from build123d import *

# Parameters (mm, degrees)
SKETCH1_W           = 2.9718
SKETCH1_H           = 25.1968
BOSS_EXTRUDE1_DEPTH = 3.175


with BuildPart() as part:
    # Sketch1 → Boss-Extrude1 (new body)
    with BuildSketch(Plane(origin=(0, 0, 0), x_dir=(1, 0, 0), z_dir=(0, 1, 0))):
        Polygon((-137.987314286, 58.785125), (-151.391257143, 58.785125), (-151.391257143, 61.960125), (-164.294457143, 61.960125), (-164.294457143, 58.785125), (-177.6984, 58.785125), (-177.6984, 61.960125), (-190.6016, 61.960125), (-190.6016, 58.785125), (-203.3016, 58.785125), (-203.3016, -58.785125), (-190.6016, -58.785125), (-190.6016, -61.960125), (-177.6984, -61.960125), (-177.6984, -58.785125), (-164.294457143, -58.785125), (-164.294457143, -61.960125), (-151.391257143, -61.960125), (-151.391257143, -58.785125), (-137.987314286, -58.785125), (-137.987314286, -61.960125), (-125.084114286, -61.960125), (-125.084114286, -58.785125), (-111.680171429, -58.785125), (-111.680171429, -61.960125), (-98.776971429, -61.960125), (-98.776971429, -58.785125), (-85.373028571, -58.785125), (-85.373028571, -61.960125), (-72.469828571, -61.960125), (-72.469828571, -58.785125), (-59.065885714, -58.785125), (-59.065885714, -61.960125), (-46.162685714, -61.960125), (-46.162685714, -58.785125), (-32.758742857, -58.785125), (-32.758742857, -61.960125), (-19.855542857, -61.960125), (-19.855542857, -58.785125), (-6.4516, -58.785125), (-6.4516, -61.960125), (6.4516, -61.960125), (6.4516, -58.785125), (19.855542857, -58.785125), (19.855542857, -61.960125), (32.758742857, -61.960125), (32.758742857, -58.785125), (46.162685714, -58.785125), (46.162685714, -61.960125), (59.065885714, -61.960125), (59.065885714, -58.785125), (72.469828571, -58.785125), (72.469828571, -61.960125), (85.373028571, -61.960125), (85.373028571, -58.785125), (98.776971429, -58.785125), (98.776971429, -61.960125), (111.680171429, -61.960125), (111.680171429, -58.785125), (125.084114286, -58.785125), (125.084114286, -61.960125), (137.987314286, -61.960125), (137.987314286, -58.785125), (151.391257143, -58.785125), (151.391257143, -61.960125), (164.294457143, -61.960125), (164.294457143, -58.785125), (177.6984, -58.785125), (177.6984, -61.960125), (190.6016, -61.960125), (190.6016, -58.785125), (203.3016, -58.785125), (203.3016, 58.785125), (190.6016, 58.785125), (190.6016, 61.960125), (177.6984, 61.960125), (177.6984, 58.785125), (164.294457143, 58.785125), (164.294457143, 61.960125), (151.391257143, 61.960125), (151.391257143, 58.785125), (137.987314286, 58.785125), (137.987314286, 61.960125), (125.084114286, 61.960125), (125.084114286, 58.785125), (111.680171429, 58.785125), (111.680171429, 61.960125), (98.776971429, 61.960125), (98.776971429, 58.785125), (85.373028571, 58.785125), (85.373028571, 61.960125), (72.469828571, 61.960125), (72.469828571, 58.785125), (59.065885714, 58.785125), (59.065885714, 61.960125), (46.162685714, 61.960125), (46.162685714, 58.785125), (32.758742857, 58.785125), (32.758742857, 61.960125), (19.855542857, 61.960125), (19.855542857, 58.785125), (6.4516, 58.785125), (6.4516, 61.960125), (-6.4516, 61.960125), (-6.4516, 58.785125), (-19.855542857, 58.785125), (-19.855542857, 61.960125), (-32.758742857, 61.960125), (-32.758742857, 58.785125), (-46.162685714, 58.785125), (-46.162685714, 61.960125), (-59.065885714, 61.960125), (-59.065885714, 58.785125), (-72.469828571, 58.785125), (-72.469828571, 61.960125), (-85.373028571, 61.960125), (-85.373028571, 58.785125), (-98.776971429, 58.785125), (-98.776971429, 61.960125), (-111.680171429, 61.960125), (-111.680171429, 58.785125), (-125.084114286, 58.785125), (-125.084114286, 61.960125), (-137.987314286, 61.960125), align=None)
        with Locations((-198.4375, 25.4)):
            Rectangle(SKETCH1_W, SKETCH1_H, mode=Mode.SUBTRACT)
        with Locations((-198.4375, -25.4)):
            Rectangle(SKETCH1_W, SKETCH1_H, mode=Mode.SUBTRACT)
        with Locations((198.4375, 25.4)):
            Rectangle(SKETCH1_W, SKETCH1_H, mode=Mode.SUBTRACT)
        with Locations((198.4375, -25.4)):
            Rectangle(SKETCH1_W, SKETCH1_H, mode=Mode.SUBTRACT)
    extrude(amount=BOSS_EXTRUDE1_DEPTH)


solid = part.part
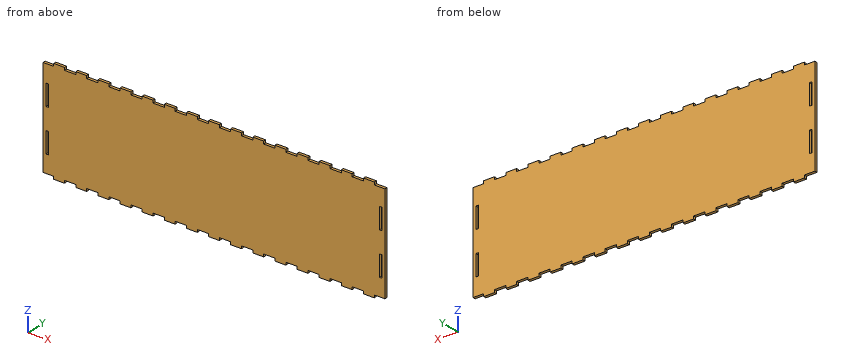
Source: CAD feature listing. Evaluate the final solid. Frame: model axes, mm. Round coordinates to 2 decimals unless told otherwise and drop trailing zeros. Loops run counter-clockwise (first coordinate to the right, second up) from the corner with the lowest first, then second, coordinate; pieces in that order, holes last. Notation, with made-up numbers: (65, -11.75) -> (112, -11.75) arc R14 ccw to (112, -4.75) -> close; hole circle Ø10 at (68.25, 40.25). An arc over 180 degrees is marked (long way). Answer as a JSON object with one key per item and string values. Group by question number.
Q1. Section query A-A (y = 1.75). State how many separate pieces and enclosed holes the cut face has, plus the area to 3 significant figures.
Q2. Contact query for flat-ended pins moving along their axis: P1, Ø1, axis at y = 1.5, z = 60, coming from the +X side; P2, Ø0.9, axis at x = -199, y = 2, coming from the -Z side; P3, Ø1.6, axis at x = 63.5, y = 2, coming from the +Z side. Output: stop coordinate, or through.
Q3. Section query B-B (x = -171.5). Output: boundary loops of the cut face in (y, z) (3 decimals).
Q4. Ray query, line 1 (X direction, y = 1.5, z = -25); line 2 (Z direction, x = 34, y = 3). Return the intervals inside material, ascending. Write a range as from..to.
Completed:
{
 "1": {"separate pieces": "1", "enclosed holes": "4", "area": "48,700 mm²"},
 "2": {"P1": "x = 190.6", "P2": "z = -58.79", "P3": "z = 58.79"},
 "3": {"outline": "(0, -58.785) -> (3.175, -58.785) -> (3.175, 58.785) -> (0, 58.785) -> close"},
 "4": {"line 1": "-203.3..-199.92, -196.95..196.95, 199.92..203.3", "line 2": "-58.79..58.79"}
}
